Study the drawing (mm; zero at the part's minimum x, y, z) and answer. Round coordinates to 2 decimals unless told otherwise and drop trailing zeros. Loops run counter-clockwise (first coordinate to the right, second up) from the corner with the lowest first, then second, coordinate; pieces in that order, holes last. Notation, with made-up numbers: (-22, -35.75) -> (17, -35.75) arc R23 cw to (17, -23.75) -> close; hole circle Ø3 at (35, 77.25). An arc over 180 degrees is marked (long way). Use one line per item in the form item = value.
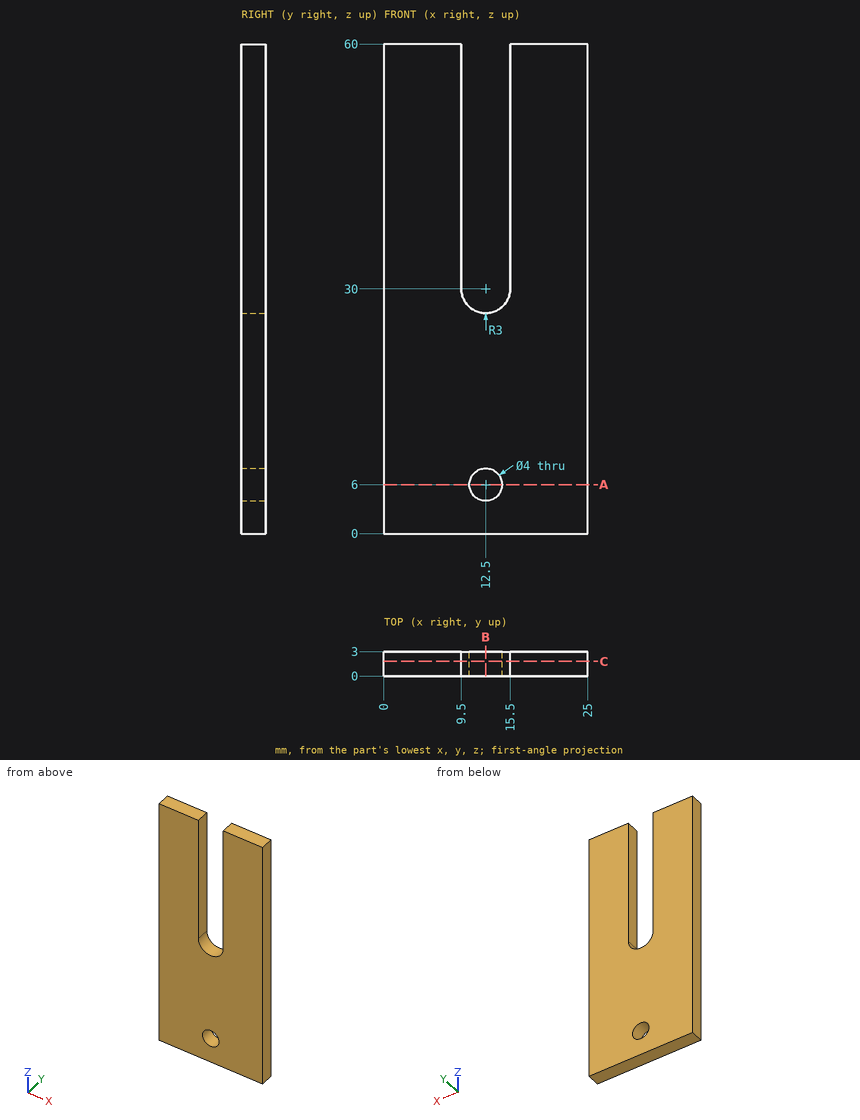
(1) Given P1, Ø1.5, axis at y = 2, z = 50, coming from the -X side, flat-ended and moving along its own axis, determine where the tip first touches the part or whether it passes through.
Completed:
P1 = 0
(2) Find section C-C, the plane y = 1.8. Write down the section's boundary in (x, z), then the cut area to 3 significant figures.
Completed:
outline = (0, 0) -> (25, 0) -> (25, 60) -> (15.5, 60) -> (15.5, 30) arc R3 cw to (9.5, 30) -> (9.5, 60) -> (0, 60) -> close; hole circle Ø4 at (12.5, 6)
area = 1,290 mm2
(3) Consider L1, parallel to X at y = 0.6, z = 6; L2, parallel to X at y = 1.5, z = 34; L3, parallel to Z at x = 12.5, y = 1.8. Determine where each line is inside the solid, lowest interval first.
Completed:
L1 = 0 to 10.5, 14.5 to 25
L2 = 0 to 9.5, 15.5 to 25
L3 = 0 to 4, 8 to 27
(4) Find section A-A, the plane z = 6. Write down the section's boundary in (x, y), then the cut area to 3 significant figures.
Completed:
outline = (0, 0) -> (10.5, 0) -> (10.5, 3) -> (0, 3) -> close; (14.5, 0) -> (25, 0) -> (25, 3) -> (14.5, 3) -> close
area = 63.0 mm2
(5) Find section B-B, the plane x = 12.5. Write down the section's boundary in (y, z), then the cut area to 3 significant figures.
Completed:
outline = (0, 0) -> (3, 0) -> (3, 4) -> (0, 4) -> close; (0, 8) -> (3, 8) -> (3, 27) -> (0, 27) -> close
area = 69.0 mm2
